```python
from build123d import *

# Parameters (mm, degrees)
SKETCH_1_W           = 15
SKETCH_1_H           = 15
EXTRUDE_1_DEPTH      = 2
SKETCH_2_W           = 4
SKETCH_2_H           = 8
CUT_EXTRUDE_1_DEPTH  = 1
EXTRUDE_2_DEPTH      = 3.5
EXTRUDE_2_DEPTH_BACK = 3.5
FILLET_1_R           = 0.1
FILLET_2_R           = 0.2


with BuildPart() as part:
    # 草图1 → 凸台-拉伸1 (new body)
    with BuildSketch(Plane(origin=(0, 0, 0), x_dir=(1, 0, 0), z_dir=(0, 1, 0))):
        Rectangle(SKETCH_1_W, SKETCH_1_H)
    extrude(amount=EXTRUDE_1_DEPTH)

    # 草图2 → 切除-拉伸1 (cut)
    with BuildSketch(Plane(origin=(0, 2, 0), x_dir=(1, 0, 0), z_dir=(0, 1, 0))):
        Rectangle(SKETCH_2_W, SKETCH_2_H)
    extrude(amount=-CUT_EXTRUDE_1_DEPTH, mode=Mode.SUBTRACT)

    # 草图3 → 凸台-拉伸2 (add, two sides: drawn at the far end of the back side and taken through both)
    with BuildSketch(Plane.XY.offset(-EXTRUDE_2_DEPTH_BACK)):
        with BuildLine():
            Line((-0.5, 1), (-1.5, 1))
            Line((-1.5, 1), (-1.5, 2.677124344))
            ThreePointArc((-1.5, 2.677124344), (-1.780042303, 3.088161527), (-1.95, 3.555590279))
            Line((-1.95, 3.555590279), (-1.95, 4))
            Line((-1.95, 4), (-1.591910703, 4))
            Line((-1.591910703, 4), (-0.5, 1))
        make_face()
        with BuildLine():
            Line((1.591910703, 4), (1.95, 4))
            Line((1.95, 4), (1.95, 3.555590279))
            ThreePointArc((1.95, 3.555590279), (1.780042303, 3.088161527), (1.5, 2.677124344))
            Line((1.5, 2.677124344), (1.5, 1))
            Line((1.5, 1), (0.5, 1))
            Line((0.5, 1), (1.591910703, 4))
        make_face()
    extrude(amount=EXTRUDE_2_DEPTH + EXTRUDE_2_DEPTH_BACK)

    # 圆角1
    fillet_1_edges = [part.edges().sort_by_distance(p)[0] for p in [
        (-1.95, 4, 0),
        (1.95, 4, 0),
    ]]
    fillet(fillet_1_edges, radius=FILLET_1_R)

    # 圆角2
    fillet_2_edges = [part.edges().sort_by_distance(p)[0] for p in [
        (7.5, 0, 0),
        (0, 0, 7.5),
        (-7.5, 0, 0),
        (0, 0, -7.5),
        (7.5, 1, -7.5),
        (7.5, 1, 7.5),
        (-7.5, 1, 7.5),
        (-7.5, 1, -7.5),
    ]]
    fillet(fillet_2_edges, radius=FILLET_2_R)


solid = part.part
```
Read the model definition and answer for the solid it produces. Units are mm, in the model's axes. A direction names the side the tool comes from. Give positions to 0.01 mm unless a question says otherwise; leave off trailing zeros. Order: outer loops, then holes, each group sorted by start corner. A loop starts at its lowest first (then second) coordinate and runs counter-clockwise, first axis right, second up.
(1) Given pin 1 (0.7 mm diameter, centred on x = 1, y = 2.5, fed in from +Z), flat-ended and moving along its own axis, determine where the tip first touches the part or whether it passes through.
(2) Straight lines are drawn through the part: L1, parallel to X at y = 1.65, z = 0.25; L2, parallel to X at y = 1.85, z = 0.5; L3, parallel to Y at x = -4.75, z = 5.75. For each, find the intervals that lie inside material, in ascending order.
(3) Find section D-D (y = 2.35). Give the vertices of the cut face in (x, z).
(4) Find section B-B (x = 3.75). Give the vertices of the cut face in (y, z), plus the area to 3 significant figures.
(5) For faces 4 (the cylindrical face through (-1.777, 3.082, -0.049)), 5 (the cylindrical face through (1.78, 3.09, -0.05)), 6 (the flat face through (-1.2, 2.2, -3.5)), 7 (the flat face through (1.5, 2, 0)), determine the directions among +Z, -Z, +X, -X, +Y, -Y from which every point of the face is accessible in a straight line to the end or side of a thin tool.
(6) For a pull along Y with two mould halves and no side action, classify faces 1 (the flat face through (-1.5, 2, 0)), 2 (the flat face through (0, 1, 7.5)), 3 (the flat face through (-1.054, 2.521, -0.049)) as released by +Y, released by -Y, zero draft, split by the parting line, or undercut.
(7) Find section C-C (z = -1.5). Give the vertices of the cut face in (x, y), plus the area to 3 significant figures.
(8) Find section A-A (y = 1.4). Give the vertices of the cut face in (x, z).
Result sheet:
1. pin 1: stops at z = 3.5
2. L1: x = -7.5 to -2, -1.5 to -0.74, 0.74 to 1.5, 2 to 7.5
2. L2: x = -7.5 to -2, -1.5 to -0.81, 0.81 to 1.5, 2 to 7.5
2. L3: y = 0 to 2
3. outline: (-1.5, -3.5) - (-0.99, -3.5) - (-0.99, 3.5) - (-1.5, 3.5) - close; (0.99, -3.5) - (1.5, -3.5) - (1.5, 3.5) - (0.99, 3.5) - close
4. outline: (0, -7.3) arc R0.2 ccw to (0.2, -7.5) - (2, -7.5) - (2, 7.5) - (0.2, 7.5) arc R0.2 ccw to (0, 7.3) - close
4. area: 30.0 mm2
5. face 4: +Z, -Z, -X
5. face 5: +Z, -Z, +X
5. face 6: +Y
5. face 7: none
6. face 1: undercut
6. face 2: zero draft
6. face 3: released by +Y
7. outline: (-7.5, 0.2) arc R0.2 ccw to (-7.3, 0) - (7.3, 0) arc R0.2 ccw to (7.5, 0.2) - (7.5, 2) - (2, 2) - (2, 1) - (1.5, 1) - (1.5, 2.68) arc R2 ccw to (1.95, 3.56) - (1.95, 3.9) arc R0.1 ccw to (1.85, 4) - (1.59, 4) - (0.5, 1) - (-0.5, 1) - (-1.59, 4) - (-1.85, 4) arc R0.1 ccw to (-1.95, 3.9) - (-1.95, 3.56) arc R2 ccw to (-1.5, 2.68) - (-1.5, 1) - (-2, 1) - (-2, 2) - (-7.5, 2) - close
7. area: 29.6 mm2
8. outline: (-7.5, -7.3) arc R0.2 ccw to (-7.3, -7.5) - (7.3, -7.5) arc R0.2 ccw to (7.5, -7.3) - (7.5, 7.3) arc R0.2 ccw to (7.3, 7.5) - (-7.3, 7.5) arc R0.2 ccw to (-7.5, 7.3) - close; (-1.5, -3.5) - (-0.65, -3.5) - (-0.65, 3.5) - (-1.5, 3.5) - close; (0.65, -3.5) - (1.5, -3.5) - (1.5, 3.5) - (0.65, 3.5) - close; hole (-2, -4) - (2, -4) - (2, 4) - (-2, 4) - close
